Source: CAD feature listing. Evaluate the final solid. Frame: model axes, mm. A direction names the side the tool comes from. Give positions to 0.01 mm unless a question says otherwise; leave off trailing zeros. Order: outer loops, then holes, each group sorted by start corner. A loop starts at its lowest first (then second) coordinate and runs counter-clockwise, first axis right, second up.
```python
from build123d import *

# Parameters (mm, degrees)
F0_W      = 25.4
F0_H      = 25.4
F1_DEPTH  = 5.08
F2_W      = 20.32
F2_H      = 20.32
F3_DEPTH  = 38.1
F4_W      = 12.7
F4_H      = 12.7
F5_DEPTH  = 7.62
F6_W      = 10.16
F6_H      = 10.16
F7_DEPTH  = 25.4
F8_W      = 5.08
F8_H      = 5.08
F9_DEPTH  = 25.4
F10_W     = 10.16
F10_H     = 10.16
F11_DEPTH = 25.4
F12_W     = 2.54
F12_H     = 2.54
F13_DEPTH = 5.08


with BuildPart() as f1:
    # F0 (on Top) → F1 (new body)
    with BuildSketch(Plane.XY):
        with Locations((12.7, -12.7)):
            Rectangle(F0_W, F0_H)
    extrude(amount=F1_DEPTH)

    # F2 (on face) → F3 (join)
    with BuildSketch(Plane.XY.offset(5.08)):
        with Locations((12.7, -12.7)):
            Rectangle(F2_W, F2_H)
    extrude(amount=F3_DEPTH)

    # F4 (on face) → F5 (cut)
    with BuildSketch(Plane.XY.offset(43.18)):
        with Locations((12.7, -12.7)):
            Rectangle(F4_W, F4_H)
    extrude(amount=-F5_DEPTH, mode=Mode.SUBTRACT)

    # F6 (on face) → F7 (cut)
    with BuildSketch(Plane.YZ.offset(22.86)):
        with Locations((-12.7, 25.4)):
            Rectangle(F6_W, F6_H)
    extrude(amount=-F7_DEPTH, mode=Mode.SUBTRACT)

    # F8 (on face) → F9 (cut)
    with BuildSketch(Plane.XY.offset(35.56)):
        with Locations((12.7, -12.7)):
            Rectangle(F8_W, F8_H)
    extrude(amount=-F9_DEPTH, mode=Mode.SUBTRACT)

    # F10 (on face) → F11 (cut)
    with BuildSketch(Plane.XZ.offset(22.86)):
        with Locations((12.7, 25.4)):
            Rectangle(F10_W, F10_H)
    extrude(amount=-F11_DEPTH, mode=Mode.SUBTRACT)

    # F12 (on face) → F13 (cut)
    with BuildSketch(Plane.XY.offset(43.18)):
        with Locations((20.955, -4.445)):
            Rectangle(F12_W, F12_H)
        with Locations((4.445, -4.445)):
            Rectangle(F12_W, F12_H)
        with Locations((4.445, -20.955)):
            Rectangle(F12_W, F12_H)
        with Locations((20.955, -20.955)):
            Rectangle(F12_W, F12_H)
    extrude(amount=-F13_DEPTH, mode=Mode.SUBTRACT)


solid = f1.part
```
1) Section query C-C, the plane x = 4. Return the cut outline in (y, z) (3 decimals), and give its area (3 significant figures).
Report:
outline: (-25.4, 0) - (0, 0) - (0, 5.08) - (-2.54, 5.08) - (-2.54, 43.18) - (-3.175, 43.18) - (-3.175, 38.1) - (-5.715, 38.1) - (-5.715, 43.18) - (-19.685, 43.18) - (-19.685, 38.1) - (-22.225, 38.1) - (-22.225, 43.18) - (-22.86, 43.18) - (-22.86, 5.08) - (-25.4, 5.08) - close; hole (-17.78, 20.32) - (-7.62, 20.32) - (-7.62, 30.48) - (-17.78, 30.48) - close
area: 774 mm2
2) Section query A-A, the plane y = -14. Return the cut outline in (x, z), and give its area (3 significant figures).
Report:
outline: (0, 0) - (25.4, 0) - (25.4, 5.08) - (22.86, 5.08) - (22.86, 20.32) - (15.24, 20.32) - (15.24, 10.16) - (10.16, 10.16) - (10.16, 20.32) - (2.54, 20.32) - (2.54, 5.08) - (0, 5.08) - close; (2.54, 30.48) - (10.16, 30.48) - (10.16, 35.56) - (6.35, 35.56) - (6.35, 43.18) - (2.54, 43.18) - close; (15.24, 30.48) - (22.86, 30.48) - (22.86, 43.18) - (19.05, 43.18) - (19.05, 35.56) - (15.24, 35.56) - close
area: 523 mm2
3) Material intervals for L1, parallel to Z at x = 16.75, y = -11; L2, parallel to Y at x = 13.5, z = 13; L3, parallel to X at y = -20.5, z = 30, sorted ascending.
Report:
L1: z = 0 to 20.32, 30.48 to 35.56
L2: y = -22.86 to -15.24, -10.16 to -2.54
L3: x = 2.54 to 7.62, 17.78 to 22.86
4) Reachability of faces 1 (the flat face through (13, -2.54, 20)), 2 (the flat face through (4, -3.175, 41)), 3 (the flat face through (13, 0, 3)) from +Z, -Z, +X, -X, +Y, -Y: full face, straight path, thin tool, end or side. Return the list, or none.
Report:
face 1: +Z, +X, -X, +Y
face 2: +Z
face 3: +Z, -Z, +X, -X, +Y
5) Section query D-D, the plane y = -21. Return the cut outline in (x, z) (3 decimals).
Report:
outline: (0, 0) - (25.4, 0) - (25.4, 5.08) - (22.86, 5.08) - (22.86, 43.18) - (22.225, 43.18) - (22.225, 38.1) - (19.685, 38.1) - (19.685, 43.18) - (5.715, 43.18) - (5.715, 38.1) - (3.175, 38.1) - (3.175, 43.18) - (2.54, 43.18) - (2.54, 5.08) - (0, 5.08) - close; hole (7.62, 20.32) - (17.78, 20.32) - (17.78, 30.48) - (7.62, 30.48) - close
6) Draft query along Z for faces 4 (the flat face through (17.78, -5, 25)), 5 (the flat face through (6, -13, 43.18)), 6 (the flat face through (13, -15.24, 15)). Return one class per face: +Z half, -Z half, draft (parallel to the pull), parting line (faces both ways), or undercut.
Report:
face 4: undercut
face 5: +Z half
face 6: draft
7) Pin query (flat end, axial travel): pin 1 (8 mm diameter, centred on x = 8.5, z = 12.5, fed in from -Y); pin 2 (2 mm diameter, centred on x = 4, y = -4.5, fed in from +Z); pin 3 (5.5 mm diameter, centred on y = -13.5, z = 33, fed in from -X); pin 4 (4 mm diameter, centred on y = -21.5, z = 25, fed in from +X). Return the tip coordinate at first contact, or that it passes through.
Report:
pin 1: stops at y = -22.86
pin 2: stops at z = 43.18
pin 3: stops at x = 2.54
pin 4: stops at x = 22.86
8) Section query B-B, the plane z = 21. Return the cut outline in (x, y), and give its area (3 significant figures).
Report:
outline: (2.54, -22.86) - (7.62, -22.86) - (7.62, -17.78) - (2.54, -17.78) - close; (2.54, -7.62) - (7.62, -7.62) - (7.62, -2.54) - (2.54, -2.54) - close; (17.78, -22.86) - (22.86, -22.86) - (22.86, -17.78) - (17.78, -17.78) - close; (17.78, -7.62) - (22.86, -7.62) - (22.86, -2.54) - (17.78, -2.54) - close
area: 103 mm2
